from build123d import *

# Parameters (mm, degrees)
SKETCH1_W           = 150
SKETCH1_H           = 25
BOSS_EXTRUDE1_DEPTH = 3
SKETCH2_W           = 12
SKETCH2_H           = 25
BOSS_EXTRUDE2_DEPTH = 12
SKETCH4_R           = 1.625
CUT_EXTRUDE1_DEPTH  = 153.541797551
SKETCH5_W           = 13
SKETCH5_H           = 22
CUT_EXTRUDE2_DEPTH  = 153.807067899


with BuildPart() as part:
    # Sketch1 → Boss-Extrude1 (new body)
    with BuildSketch(Plane(origin=(0, 0, 0), x_dir=(1, 0, 0), z_dir=(0, 1, 0))):
        with Locations((75, 12.5)):
            Rectangle(SKETCH1_W, SKETCH1_H)
    extrude(amount=BOSS_EXTRUDE1_DEPTH)

    # Sketch2 → Boss-Extrude2 (add)
    with BuildSketch(Plane.XZ):
        with Locations((6, -12.5)):
            Rectangle(SKETCH2_W, SKETCH2_H)
        with Locations((144, -12.5)):
            Rectangle(SKETCH2_W, SKETCH2_H)
    extrude(amount=BOSS_EXTRUDE2_DEPTH)

    # Sketch4 → Cut-Extrude1 (cut, through all)
    with BuildSketch(Plane.XY):
        with Locations((6, -6)):
            Circle(SKETCH4_R)
        with Locations(Location((144, -6, 0), (0, 0, 180))):
            Circle(SKETCH4_R)
    extrude(amount=-CUT_EXTRUDE1_DEPTH, mode=Mode.SUBTRACT)

    # Sketch5 → Cut-Extrude2 (cut, through all)
    with BuildSketch(Plane(origin=(0, 3, 0), x_dir=(1, 0, 0), z_dir=(0, 1, 0))):
        with Locations((143.5, 11)):
            Rectangle(SKETCH5_W, SKETCH5_H)
    extrude(amount=-CUT_EXTRUDE2_DEPTH, mode=Mode.SUBTRACT)


solid = part.part
Geometry: final body of the model. Coordinates: model frame, mm. A direction names the side the tool comes from. Round coordinates to 2 decimals unless told otherwise and drop trailing zeros. Write each loop counter-clockwise with the first axis right and the second up, starting at its lowest first coordinate (ties: lowest second). Pieces come first, ordered by that corner, then holes. Notation, with made-up numbers: M 34,55 L 92,55 A17 cw 92,84 Z; hole C 42,35 d7. An arc over 180 degrees is marked long. Write item = value, one per line.
Item 1: Material intervals for line 1 along Y through (x, z) = (6, -6.5) (3 decimals); line 2 along X through (y, z) = (-10.75, -24); line 3 along X through (y, z) = (1.75, -6), sorted ascending. Write a range as [from, to].
Findings:
line_1 = [-12, -7.625], [-4.375, 3]
line_2 = [0, 12], [138, 150]
line_3 = [0, 137]
Item 2: Section query D-D on x = 6. Return loops of the section in (y, z) (3 decimals).
Findings:
outline = M -12,-25 L -7.625,-25 L -7.625,0 L -12,0 Z; M -4.375,-25 L 3,-25 L 3,0 L -4.375,0 Z
Item 3: Pin query (flat end, axial travel): P1, Ø4, axis at x = 140.5, y = -7, coming from the +Z side; P2, Ø12, axis at x = 39.5, z = -6.5, coming from the -Y side; P3, Ø6, axis at y = -8, z = -14.5, coming from the +X side. Return the tip coordinate at first contact, or that it passes through.
Findings:
P1 = -22
P2 = 0
P3 = 12
Item 4: Section query A-A on y = -6. Return loops of the section in (x, z) (3 decimals), then the cut area to 3 significant figures.
Findings:
outline = M 0,-25 L 4.375,-25 L 4.375,0 L 0,0 Z; M 7.625,-25 L 12,-25 L 12,0 L 7.625,0 Z; M 138,-25 L 142.375,-25 L 142.375,-22 L 138,-22 Z; M 145.625,-25 L 150,-25 L 150,-22 L 145.625,-22 Z
area = 245 mm^2
Item 5: Section query C-C on x = 144. Return loops of the section in (y, z) (3 decimals), then the cut area to 4 significant figures.
Findings:
outline = M -12,-25 L -7.625,-25 L -7.625,-22 L -12,-22 Z; M -4.375,-25 L 3,-25 L 3,-22 L -4.375,-22 Z
area = 35.25 mm^2
Item 6: Access query for faces 1 (the face through (137, 2, -11)), 2 (the face through (138, -6, -24)), 3 (the face through (74, 1, -25)). Directions: +Z, -Z, +X, -X, +Y, -Y. A direction counts if a zero-diameter tool reaches every point of the face in a straight line with its end or side. Return the directions, or none.
Findings:
face_1 = +Z, +X, +Y, -Y
face_2 = +Z, -Z, -Y
face_3 = -Z, +X, -X, +Y, -Y
Item 7: Section query B-B on z = -20.25. Return loops of the section in (x, y) (3 decimals).
Findings:
outline = M 0,-12 L 12,-12 L 12,0 L 137,0 L 137,3 L 0,3 Z; hole C 6,-6 d3.25
Item 8: Pull-direction query (X, two-part tool) for faces 4 (the face through (4.802, -4.902, -12.325)), 5 (the face through (145.623, -6.071, -23.479)), 6 (the face through (53, 1, 0)), 7 (the face through (0, -4, -13)); classes: pulls with the +X half, pulls with the -X half, needs draft (parallel to the pull), parting line crosses it, or undercut.
Findings:
face_4 = undercut
face_5 = undercut
face_6 = needs draft
face_7 = pulls with the -X half
